Geometry check sheet. Reference: the model listing, model coordinates, mm. Face numbers are marked on the shaded views. A direction names the side the tool comes from. Coordinates: 2 decimals unless noted, no trailing zeros. Loops run counter-clockwise (first coordinate to the right, second up) from the corner with the lowest first, then second, coordinate; pieces in that order, holes last.
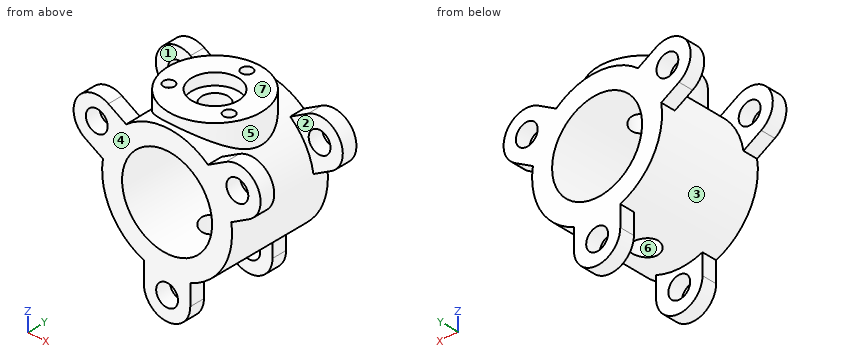
from build123d import *

# Parameters (mm, degrees)
SKETCH1_R                   = 140
SKETCH1_R_2                 = 97
BOSS_EXTRUDE1_DEPTH         = 225
SKETCH2_R                   = 23.5
BOSS_EXTRUDE2_DEPTH         = 32
CIRPATTERN1_COUNT           = 3
LPATTERN2_COUNT             = 2
LPATTERN2_PITCH             = 193
CIRPATTERN2_COPY_1_SKETCH_R = 23.5
CIRPATTERN2_COPY_1_DEPTH    = 32
CIRPATTERN2_COPY_2_SKETCH_R = 23.5
CIRPATTERN2_COPY_2_DEPTH    = 32
CIRPATTERN2_COPY_3_SKETCH_R = 23.5
CIRPATTERN2_COPY_3_DEPTH    = 32
CIRPATTERN2_COPY_4_SKETCH_R = 23.5
CIRPATTERN2_COPY_4_DEPTH    = 32
BOSS_EXTRUDE3_REACH         = 387
SKETCH3_R                   = 100
SKETCH4_R                   = 28
CUT_EXTRUDE1_DEPTH          = 386
SKETCH5_R                   = 50
CUT_EXTRUDE2_DEPTH          = 25
SKETCH6_R                   = 12
CUT_EXTRUDE3_DEPTH          = 15


with BuildPart() as part:
    # Sketch1 → Boss-Extrude1 (new body)
    with BuildSketch(Plane(origin=(0, 0, 0), x_dir=(1, 0, 0), z_dir=(0, 1, 0))):
        Circle(SKETCH1_R)
        Circle(SKETCH1_R_2, mode=Mode.SUBTRACT)
    extrude(amount=BOSS_EXTRUDE1_DEPTH)

    # Sketch2 → Boss-Extrude2 (add)
    with BuildSketch(Plane(origin=(0, 225, 0), x_dir=(1, 0, 0), z_dir=(0, 1, 0))):
        with BuildLine():
            Line((-50, 130.766968306), (-50, 175))
            ThreePointArc((-50, 175), (0, 225), (50, 175))
            Line((50, 175), (50, 130.766968306))
            ThreePointArc((50, 130.766968306), (0, 140), (-50, 130.766968306))
        make_face()
        with Locations((0, 175)):
            Circle(SKETCH2_R, mode=Mode.SUBTRACT)
    boss_extrude2 = extrude(amount=-BOSS_EXTRUDE2_DEPTH)

    # CirPattern1: Boss-Extrude2 ×3 about axis
    cirpattern1_axis = Axis((0, 0, 0), (0, 1, 0))
    for i in range(1, CIRPATTERN1_COUNT):
        add(boss_extrude2.rotate(cirpattern1_axis, i * 360 / CIRPATTERN1_COUNT))

    # LPattern2: Boss-Extrude2 ×2
    with Locations(*[(0, -i * LPATTERN2_PITCH, 0) for i in range(1, LPATTERN2_COUNT)]):
        add(boss_extrude2)

    # CirPattern2 copy 1 sketch → CirPattern2 copy 1 (add)
    with BuildSketch(Plane(origin=(0, 32, 0), x_dir=(-0.5, 0, -0.866025404), z_dir=(0, 1, 0))):
        with BuildLine():
            Line((-50, 130.766968306), (-50, 175))
            ThreePointArc((-50, 175), (0, 225), (50, 175))
            Line((50, 175), (50, 130.766968306))
            ThreePointArc((50, 130.766968306), (0, 140), (-50, 130.766968306))
        make_face()
        with Locations((0, 175)):
            Circle(CIRPATTERN2_COPY_1_SKETCH_R, mode=Mode.SUBTRACT)
    extrude(amount=-CIRPATTERN2_COPY_1_DEPTH)

    # CirPattern2 copy 2 sketch → CirPattern2 copy 2 (add)
    with BuildSketch(Plane(origin=(0, 32, 0), x_dir=(-0.5, 0, 0.866025404), z_dir=(0, 1, 0))):
        with BuildLine():
            Line((-50, 130.766968306), (-50, 175))
            ThreePointArc((-50, 175), (0, 225), (50, 175))
            Line((50, 175), (50, 130.766968306))
            ThreePointArc((50, 130.766968306), (0, 140), (-50, 130.766968306))
        make_face()
        with Locations((0, 175)):
            Circle(CIRPATTERN2_COPY_2_SKETCH_R, mode=Mode.SUBTRACT)
    extrude(amount=-CIRPATTERN2_COPY_2_DEPTH)

    # CirPattern2 copy 3 sketch → CirPattern2 copy 3 (add)
    with BuildSketch(Plane(origin=(0, 225, 0), x_dir=(-0.5, 0, -0.866025404), z_dir=(0, 1, 0))):
        with BuildLine():
            Line((-50, 130.766968306), (-50, 175))
            ThreePointArc((-50, 175), (0, 225), (50, 175))
            Line((50, 175), (50, 130.766968306))
            ThreePointArc((50, 130.766968306), (0, 140), (-50, 130.766968306))
        make_face()
        with Locations((0, 175)):
            Circle(CIRPATTERN2_COPY_3_SKETCH_R, mode=Mode.SUBTRACT)
    extrude(amount=-CIRPATTERN2_COPY_3_DEPTH)

    # CirPattern2 copy 4 sketch → CirPattern2 copy 4 (add)
    with BuildSketch(Plane(origin=(0, 225, 0), x_dir=(-0.5, 0, 0.866025404), z_dir=(0, 1, 0))):
        with BuildLine():
            Line((-50, 130.766968306), (-50, 175))
            ThreePointArc((-50, 175), (0, 225), (50, 175))
            Line((50, 175), (50, 130.766968306))
            ThreePointArc((50, 130.766968306), (0, 140), (-50, 130.766968306))
        make_face()
        with Locations((0, 175)):
            Circle(CIRPATTERN2_COPY_4_SKETCH_R, mode=Mode.SUBTRACT)
    extrude(amount=-CIRPATTERN2_COPY_4_DEPTH)

    # Sketch3 → Boss-Extrude3 (add, up to next)
    with BuildSketch(Plane.XY.offset(160), mode=Mode.PRIVATE) as boss_extrude3_sk1:
        with Locations((0, 112.5)):
            Circle(SKETCH3_R)
    boss_extrude3_tool1 = extrude(boss_extrude3_sk1.sketch, amount=-BOSS_EXTRUDE3_REACH, mode=Mode.PRIVATE) - part.part
    add(boss_extrude3_tool1.solids().sort_by_distance((0, 112.5, 160))[0])

    # Sketch4 → Cut-Extrude1 (cut, through all)
    with BuildSketch(Plane.XY.offset(160)):
        with Locations((0, 112.5)):
            Circle(SKETCH4_R)
    extrude(amount=-CUT_EXTRUDE1_DEPTH, mode=Mode.SUBTRACT)

    # Sketch5 → Cut-Extrude2 (cut)
    with BuildSketch(Plane.XY.offset(160)):
        with Locations((0, 112.5)):
            Circle(SKETCH5_R)
    extrude(amount=-CUT_EXTRUDE2_DEPTH, mode=Mode.SUBTRACT)

    # Sketch6 → Cut-Extrude3 (cut)
    with BuildSketch(Plane.XY.offset(160)):
        with Locations((0, 187.5)):
            Circle(SKETCH6_R)
        with Locations((64.951905284, 75)):
            Circle(SKETCH6_R)
        with Locations((-64.951905284, 75)):
            Circle(SKETCH6_R)
    extrude(amount=-CUT_EXTRUDE3_DEPTH, mode=Mode.SUBTRACT)


solid = part.part
(1) Sectioned sample at A-A on x = 59.5. Record the cut outline in (y, z).
Findings:
outline: (0, -126.73) - (225, -126.73) - (225, -76.61) - (0, -76.61) - close; (0, 76.61) - (225, 76.61) - (225, 126.73) - (192.87, 126.73) - (192.87, 160) - (85.69, 160) - (85.69, 145) - (64.31, 145) - (64.31, 160) - (32.13, 160) - (32.13, 126.73) - (0, 126.73) - close
(2) Sectioned sample at B-B on y = 96. Record the cut outline in (x, z), and give its area (3 significant figures).
Findings:
outline: (-98.63, 99.36) arc R140 ccw to (-22.62, -138.16) - (-22.62, -94.33) arc R97 cw to (-22.62, 94.33) - (-22.62, 135) - (-47.2, 135) - (-47.2, 160) - (-98.63, 160) - close; (22.62, -138.16) arc R140 ccw to (98.63, 99.36) - (98.63, 160) - (47.2, 160) - (47.2, 135) - (22.62, 135) - (22.62, 94.33) arc R97 cw to (22.62, -94.33) - close
area: 32,400 mm2
(3) Draft check along X on the marked faces 6 and 7. Enter one of: +X half, -X half, draft (parallel to the pull), parting line (faces both ways), or undercut.
Findings:
face 6: undercut
face 7: draft
(4) Sectioned sample at D-D on x = 0. State how many separate pieces and enclosed holes the cut face has, and give its area (3 significant figures).
Findings:
separate pieces: 6
enclosed holes: 0
area: 18,400 mm2
(5) Scan lines: L1, parallel to Z at x = 0, y = 17; L2, parallel to Y at x = 0, z = 104.5; L3, parallel to X at y = 18, z = -175. Record each from-to range of solid material in increasing order.
Findings:
L1: z = -225 to -198.5, -151.5 to -97, 97 to 160
L2: y = 0 to 84.5, 140.5 to 225
L3: x = -50 to -23.5, 23.5 to 50
(6) Sectioned sample at C-C on z = -67. Record the cut outline in (x, y), and give its area (3 significant figures).
Findings:
outline: (-122.93, 0) - (-70.14, 0) - (-70.14, 225) - (-122.93, 225) - close; (70.14, 0) - (122.93, 0) - (122.93, 225) - (70.14, 225) - close
area: 23,800 mm2
(7) Access from +Z, -Z, +X, -X, +Y, -Y to the whole of each face (thin tool, end or side, straight path). Record for the marked faces 1, 2, 3, 4 and 5.
Findings:
face 1: +Z, -X
face 2: +Z, +X
face 3: none
face 4: +Z, -Z, +X, -X, -Y
face 5: +Z
(8) Gauge pin test, flat ends, axial feed: pin 1 Ø5 at (y, z) = (147, -64) entering from +X; pin 2 Ø7 at (x, y) = (-61, 70.5) entering from +Z; pin 3 Ø12 at (x, y) = (105, 155.5) entering from -Z. Record the tip position at first contact, or that the pin passes through.
Findings:
pin 1: stops at x = 125.77
pin 2: stops at z = 145
pin 3: stops at z = -98.99
